from build123d import *

# Parameters (mm, degrees)
BOSS_EXTRUDE1_DEPTH                  = 330.200001
BOSS_EXTRUDE1_DEPTH_BACK             = 330.200001
SKETCH3_W                            = 38.1
SKETCH3_H                            = 25.4
SKETCH3_W_2                          = 31.75
SKETCH3_H_2                          = 19.05
F_1_4_0_25_DIAMETER_HOLE2_AT_2_COUNT = 2
F_1_4_0_25_DIAMETER_HOLE2_AT_2_PITCH = 25.4
F_1_4_0_25_DIAMETER_HOLE2_AT_3_COUNT = 2
F_1_4_0_25_DIAMETER_HOLE2_AT_3_PITCH = 635.000000508
F_1_4_0_25_DIAMETER_HOLE2_AT_4_COUNT = 2
F_1_4_0_25_DIAMETER_HOLE2_AT_4_PITCH = 50.8
F_1_4_0_25_DIAMETER_HOLE2_AT_5_COUNT = 2
F_1_4_0_25_DIAMETER_HOLE2_AT_5_PITCH = 609.600000508
F_1_4_0_25_DIAMETER_HOLE3_D          = 6.35
F_13_64_0_20313_DIAMETER_HOLE1_D     = 5.159502
F_10_CLEARANCE_HOLE1_D               = 4.9784


with BuildPart() as part:
    # Sketch3 → Boss-Extrude1 (new, two sides: drawn at the far end of the back side and taken through both)
    with BuildSketch(Plane.XY.offset(-BOSS_EXTRUDE1_DEPTH_BACK)):
        Rectangle(SKETCH3_W, SKETCH3_H)
        Rectangle(SKETCH3_W_2, SKETCH3_H_2, mode=Mode.SUBTRACT)
    extrude(amount=BOSS_EXTRUDE1_DEPTH + BOSS_EXTRUDE1_DEPTH_BACK)

    # Sketch8 → 1/4 (0.25) Diameter Hole2 (revolve, cut)
    with BuildSketch(Plane(origin=(-19.05, 0, -317.500000508), x_dir=(0, 0, 1), z_dir=(0, 1, 0))):
        Polygon((0, 0), (0, 38.1), (3.9624, 38.1), (3.175, 37.194199916), (3.175, 0), align=None)
    f_1_4_0_25_diameter_hole2 = revolve(axis=Axis((-25.4, 0, -317.500000508), (1, 0, 0)), mode=Mode.SUBTRACT)

    # 1/4 (0.25) Diameter Hole2 at 2: 1/4 (0.25) Diameter Hole2 ×2
    with Locations(*[(0, 0, i * F_1_4_0_25_DIAMETER_HOLE2_AT_2_PITCH) for i in range(1, F_1_4_0_25_DIAMETER_HOLE2_AT_2_COUNT)]):
        add(f_1_4_0_25_diameter_hole2, mode=Mode.SUBTRACT)

    # 1/4 (0.25) Diameter Hole2 at 3: 1/4 (0.25) Diameter Hole2 ×2
    with Locations(*[(0, 0, i * F_1_4_0_25_DIAMETER_HOLE2_AT_3_PITCH) for i in range(1, F_1_4_0_25_DIAMETER_HOLE2_AT_3_COUNT)]):
        add(f_1_4_0_25_diameter_hole2, mode=Mode.SUBTRACT)

    # 1/4 (0.25) Diameter Hole2 at 4: 1/4 (0.25) Diameter Hole2 ×2
    with Locations(*[(0, 0, i * F_1_4_0_25_DIAMETER_HOLE2_AT_4_PITCH) for i in range(1, F_1_4_0_25_DIAMETER_HOLE2_AT_4_COUNT)]):
        add(f_1_4_0_25_diameter_hole2, mode=Mode.SUBTRACT)

    # 1/4 (0.25) Diameter Hole2 at 5: 1/4 (0.25) Diameter Hole2 ×2
    with Locations(*[(0, 0, i * F_1_4_0_25_DIAMETER_HOLE2_AT_5_PITCH) for i in range(1, F_1_4_0_25_DIAMETER_HOLE2_AT_5_COUNT)]):
        add(f_1_4_0_25_diameter_hole2, mode=Mode.SUBTRACT)

    # 1/4 (0.25) Diameter Hole3 (through all)
    with Locations(Plane(origin=(19.05, 0, 0), x_dir=(0, 0, -1), z_dir=(1, 0, 0))):
        with Locations((-266.7, 0), (-241.3, 0), (-215.9, 0), (241.300000508, 0), (215.900000508, 0), (190.500000508, 0)):
            Hole(F_1_4_0_25_DIAMETER_HOLE3_D / 2)

    # 13/64 (0.20313) Diameter Hole1 (through all)
    with Locations(Plane(origin=(19.05, 0, 0), x_dir=(0, 0, -1), z_dir=(1, 0, 0))):
        with Locations((152.400000508, 0), (-177.799999492, 0)):
            Hole(F_13_64_0_20313_DIAMETER_HOLE1_D / 2)

    # #10 Clearance Hole1 (through all)
    with Locations(Plane(origin=(19.05, 0, 0), x_dir=(0, 0, -1), z_dir=(1, 0, 0))):
        with Locations((-128.5875, 0), (-103.1875, 0), (77.787500575, 1.014e-06), (103.187500575, 1.014e-06)):
            Hole(F_10_CLEARANCE_HOLE1_D / 2)


solid = part.part
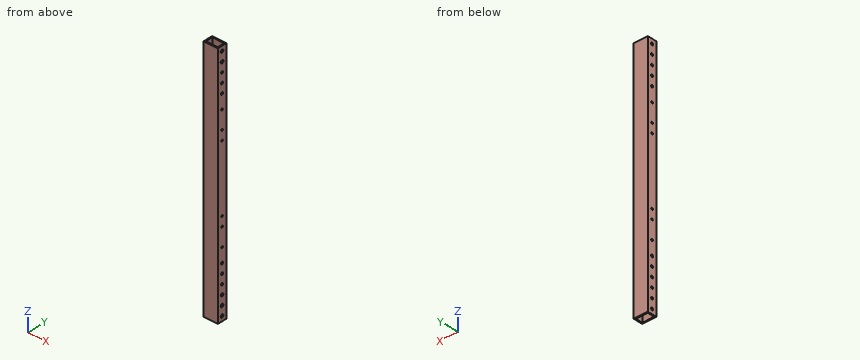
Work out the finished part from the listing and answer in its coordinate system (mm). Round coordinates to 2 decimals unless told otherwise and drop trailing zeros. Order: outer loops, then holes, each group sorted by start corner. A loop starts at its lowest first (then second) coordinate and runs counter-clockwise, first axis right, second up. Notation, with made-up numbers: M 16,7 L 21,7 A10 cw 21,14 Z; hole C -19,11 d6. An arc over 180 degrees is marked long. Put each result on its own line as item: value. Start each with the question number.
Q1. Straight lines are drawn through the part: L1, parallel to Y at x = -8, z = 205.5 (3 decimals); L2, parallel to X at y = -6.75, z = 277.5 (3 decimals); L3, parallel to Y at x = 17.1, z = -266.7 (3 decimals). For each, find the intervals that lie inside material, in ascending order. Write a range as [from, to].
Q2. Section A-A, the plane x = 0.5 is taken. Write down the section's boundary in (y, z) (3 decimals), and give its area (3 significant figures).
Q3. Flat-ended cylindrical pins translate along their axes: pin 1 (4 mm diameter, centred on x = -13.5, y = 2.5, fed in from -Z); pin 2 (6.5 mm diameter, centred on y = 0, z = -103.19, fed in from -X). Find the tip coordinate at first contact, or state that the pin passes through.
Q4. Section B-B, the plane z = -126.5 is taken. Write down the section's boundary in (x, y) (3 decimals), and give its area (3 significant figures).
Findings below:
1. L1: y = [-12.7, -9.525], [9.525, 12.7]
1. L2: x = [-19.05, -15.875], [15.875, 19.05]
1. L3: y = [-12.7, -3.175], [3.175, 12.7]
2. outline: M -12.7,-330.2 L -9.525,-330.2 L -9.525,330.2 L -12.7,330.2 Z; M 9.525,-330.2 L 12.7,-330.2 L 12.7,330.2 L 9.525,330.2 Z
2. area: 4,190 mm^2
3. pin 1: passes through
3. pin 2: stops at x = -19.05
4. outline: M -19.05,-12.7 L 19.05,-12.7 L 19.05,12.7 L -19.05,12.7 Z; hole M -15.875,-9.525 L 15.875,-9.525 L 15.875,9.525 L -15.875,9.525 Z
4. area: 363 mm^2
